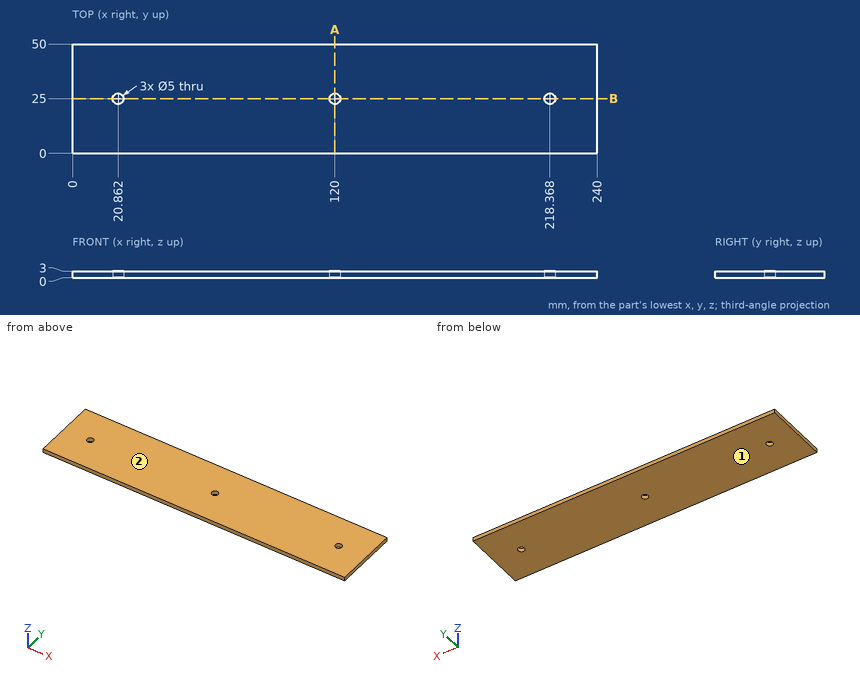
Input: dimensioned drawing with shaded views. Units: mm. Origin: part minimum x, y, z. Give positions to 0.01 mm unless a question says otherwise; leave off trailing zeros. Write each loop counter-clockwise with the first axis right and the second up, starting at its lowest first coordinate (ties: lowest second). Pieces come first, ordered by that corner, then holes.
1. Section query B-B, the plane y = 25. Return loops of the section in (x, z), then the cut area to 3 significant figures.
2. Section query A-A, the plane x = 120. Return loops of the section in (y, z), then the cut area to 3 significant figures.
3. Line query: probe 1 along Y at (x, z) = (120, 1.9); probe 2 along X at (y, z) = (25.5, 1.35). Output: solid intervals per line, ascending.
4. Pin query (flat end, axial travel): P1, Ø3, axis at x = 20.86, y = 25, coming from the +Z side. Return the tip coordinate at first contact, or that it passes through.
5. Draft query along Z for the marked faces 1 and 2. Return one class per face: released by +Z, released by -Z, zero draft, split by the parting line, or undercut.
Computed:
1. outline: (0, 0) - (18.36, 0) - (18.36, 3) - (0, 3) - close; (23.36, 0) - (117.5, 0) - (117.5, 3) - (23.36, 3) - close; (122.5, 0) - (215.87, 0) - (215.87, 3) - (122.5, 3) - close; (220.87, 0) - (240, 0) - (240, 3) - (220.87, 3) - close
1. area: 675 mm2
2. outline: (0, 0) - (22.5, 0) - (22.5, 3) - (0, 3) - close; (27.5, 0) - (50, 0) - (50, 3) - (27.5, 3) - close
2. area: 135 mm2
3. probe 1: y = 0 to 22.5, 27.5 to 50
3. probe 2: x = 0 to 18.41, 23.31 to 117.55, 122.45 to 215.92, 220.82 to 240
4. P1: passes through
5. face 1: released by -Z
5. face 2: released by +Z
